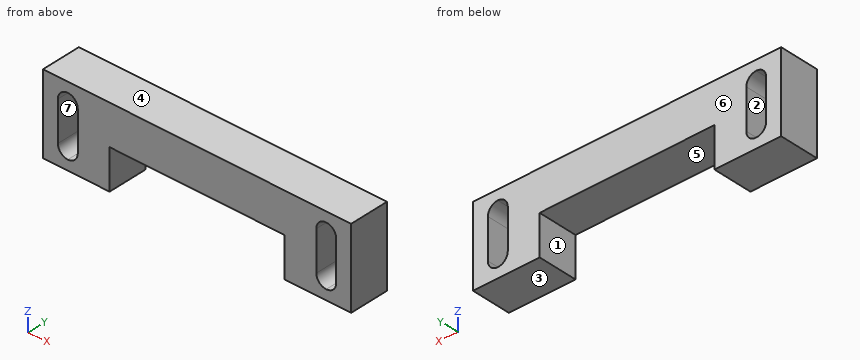
from build123d import *

# Parameters (mm, degrees)
SKETCH1_W            = 98.425
SKETCH1_H            = 12.7
BOSS_EXTRUDE1_DEPTH  = 12.7
CUT_EXTRUDE1_REACH   = 54.388
SKETCH2_W            = 6.35
SKETCH2_H            = 19.05
FILLET1_R            = 3.175
FILLET2_R            = 3.175
FILLET3_R            = 3.175
FILLET4_R            = 3.175
FILLET1_OF_MIRROR1_R = 3.175
FILLET2_OF_MIRROR1_R = 3.175
FILLET3_OF_MIRROR1_R = 3.175
FILLET4_OF_MIRROR1_R = 3.175
CUT_EXTRUDE2_REACH   = 54.388
SKETCH5_W            = 55.88
SKETCH5_H            = 12.7


with BuildPart() as part:
    # Sketch1 → Boss-Extrude1 (new, symmetric)
    with BuildSketch(Plane.XY):
        Rectangle(SKETCH1_W, SKETCH1_H)
    extrude(amount=BOSS_EXTRUDE1_DEPTH, both=True)

    # Sketch2 → Cut-Extrude1 (cut, up to next)
    with BuildSketch(Plane(origin=(0, 6.35, 0), x_dir=(1, 0, 0), z_dir=(0, 1, 0)), mode=Mode.PRIVATE) as cut_extrude1_sk1:
        with Locations((-41.275, 0)):
            Rectangle(SKETCH2_W, SKETCH2_H)
    cut_extrude1_tool1 = extrude(cut_extrude1_sk1.sketch, amount=-CUT_EXTRUDE1_REACH, mode=Mode.PRIVATE) & part.part
    cut_extrude1 = cut_extrude1_tool1.solids().sort_by_distance((-41.275, 6.35, 0))[0]
    add(cut_extrude1, mode=Mode.SUBTRACT)

    # Fillet1
    fillet1_edges = [part.edges().sort_by_distance(p)[0] for p in [
        (-44.45, 0, -9.525),
    ]]
    fillet(fillet1_edges, radius=FILLET1_R)

    # Fillet2
    fillet2_edges = [part.edges().sort_by_distance(p)[0] for p in [
        (-38.1, 0, -9.525),
    ]]
    fillet(fillet2_edges, radius=FILLET2_R - 0.0001)  # a hair under: the kernel refuses the full size

    # Fillet3
    fillet3_edges = [part.edges().sort_by_distance(p)[0] for p in [
        (-44.45, 0, 9.525),
    ]]
    fillet(fillet3_edges, radius=FILLET3_R)

    # Fillet4
    fillet4_edges = [part.edges().sort_by_distance(p)[0] for p in [
        (-38.1, 0, 9.525),
    ]]
    fillet(fillet4_edges, radius=FILLET4_R - 0.0001)  # a hair under: the kernel refuses the full size

    # Mirror1: Cut-Extrude1 across plane
    add(cut_extrude1.mirror(Plane(origin=(0, 0, 0), x_dir=(0, 0, 1), z_dir=(1, 0, 0))), mode=Mode.SUBTRACT)

    # Fillet1 of Mirror1
    fillet1_of_mirror1_edges = [part.edges().sort_by_distance(p)[0] for p in [
        (44.45, 0, -9.525),
    ]]
    fillet(fillet1_of_mirror1_edges, radius=FILLET1_OF_MIRROR1_R)

    # Fillet2 of Mirror1
    fillet2_of_mirror1_edges = [part.edges().sort_by_distance(p)[0] for p in [
        (38.1, 0, -9.525),
    ]]
    fillet(fillet2_of_mirror1_edges, radius=FILLET2_OF_MIRROR1_R - 0.0001)  # a hair under: the kernel refuses the full size

    # Fillet3 of Mirror1
    fillet3_of_mirror1_edges = [part.edges().sort_by_distance(p)[0] for p in [
        (44.45, 0, 9.525),
    ]]
    fillet(fillet3_of_mirror1_edges, radius=FILLET3_OF_MIRROR1_R)

    # Fillet4 of Mirror1
    fillet4_of_mirror1_edges = [part.edges().sort_by_distance(p)[0] for p in [
        (38.1, 0, 9.525),
    ]]
    fillet(fillet4_of_mirror1_edges, radius=FILLET4_OF_MIRROR1_R - 0.0001)  # a hair under: the kernel refuses the full size

    # Sketch5 → Cut-Extrude2 (cut, up to next)
    with BuildSketch(Plane(origin=(0, 6.35, 0), x_dir=(1, 0, 0), z_dir=(0, 1, 0)), mode=Mode.PRIVATE) as cut_extrude2_sk1:
        with Locations((0, 6.35)):
            Rectangle(SKETCH5_W, SKETCH5_H)
    cut_extrude2_tool1 = extrude(cut_extrude2_sk1.sketch, amount=-CUT_EXTRUDE2_REACH, mode=Mode.PRIVATE) & part.part
    add(cut_extrude2_tool1.solids().sort_by_distance((0, 6.35, -6.35))[0], mode=Mode.SUBTRACT)


solid = part.part
The model under review builds one solid part; all positions refer to its coordinate system, in mm. Face numbers are marked on the shaded views. A direction names the side the tool comes from. Give positions to 0.01 mm unless a question says otherwise; leave off trailing zeros. Write each loop counter-clockwise with the first axis right and the second up, starting at its lowest first coordinate (ties: lowest second). Pieces come first, ordered by that corner, then holes.
1. Add section B-B, the plane y = -3. Count the separate pieces of the cut face and the enclosed holes in it, plus the area to 3 significant figures.
2. Wall thickness on L1, parallel to X at y = 2, z = -5.25; L2, parallel to X at y = -1, z = 2; L3, parallel to X at y = 3, z = -8: over which ranges is each line inside the solid? List them lowest first.
3. Add section C-C, the plane x = -39.5. Write out the cut boundary in (y, z), plus the area to 3 significant figures.
4. Draft analysis for pull direction Z (two halves, no side actions). For the marked faces 1, 2, 3 and 4, state which applies: +Z half, -Z half, draft (parallel to the pull), parting line (faces both ways), or undercut.
5. Tool access review of the marked faces 5, 6 and 7: name each direction out of +Z, -Z, +X, -X, +Y, -Y from which nothing blocks a thin tool from reaching the whole face with its end or side.
6. Add section A-A, the plane z = -10.75. Write out the cut boundary in (x, y).
7. Add section D-D, the plane z = 8.5. Write out the cut boundary in (x, y).
Worked answers:
1. separate pieces: 1
1. enclosed holes: 2
1. area: 1,570 mm2
2. L1: x = -49.21 to -44.45, -38.1 to -27.94, 27.94 to 38.1, 44.45 to 49.21
2. L2: x = -49.21 to -44.45, -38.1 to 38.1, 44.45 to 49.21
2. L3: x = -49.21 to -43.99, -38.56 to -27.94, 27.94 to 38.56, 43.99 to 49.21
3. outline: (-6.35, -12.7) - (6.35, -12.7) - (6.35, -8.98) - (-6.35, -8.98) - close; (-6.35, 8.98) - (6.35, 8.98) - (6.35, 12.7) - (-6.35, 12.7) - close
3. area: 94.4 mm2
4. face 1: draft
4. face 2: undercut
4. face 3: -Z half
4. face 4: +Z half
5. face 5: -Z, +Y, -Y
5. face 6: +Z, -Z, +X, -X, +Y
5. face 7: +Y, -Y
6. outline: (-49.21, -6.35) - (-27.94, -6.35) - (-27.94, 6.35) - (-49.21, 6.35) - close; (27.94, -6.35) - (49.21, -6.35) - (49.21, 6.35) - (27.94, 6.35) - close
7. outline: (-49.21, -6.35) - (-43.61, -6.35) - (-43.61, 6.35) - (-49.21, 6.35) - close; (-38.94, -6.35) - (38.94, -6.35) - (38.94, 6.35) - (-38.94, 6.35) - close; (43.61, -6.35) - (49.21, -6.35) - (49.21, 6.35) - (43.61, 6.35) - close
